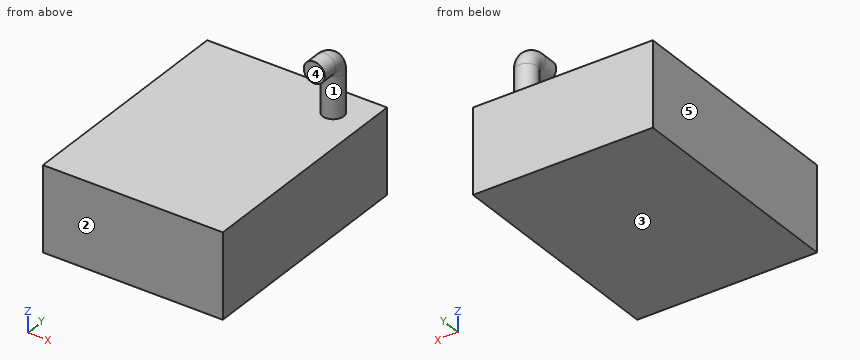
Autodesk Inventor part; units mm, degrees
ref_plane "Work Plane1" through (-215.9, 177.6349, 0) normal (0, 1, 0) x (1, 0, 0)
ref_plane "Work Plane2" through (139.7, -280.9875, 0) normal (1, 0, 0) x (0, 0, -1)
ref_plane "YZ Plane" through (0, 0, 0) normal (1, 0, 0) x (0, 1, 0)
sketch "Sketch1" plane through (0, 0, 0) normal (0, 0, 1) x (1, 0, 0)
  line L0 (215.9, -280.9875) -> (-215.9, -280.9875)
  line L1 (-215.9, -280.9875) -> (-215.9, 280.9875)
  line L2 (-215.9, 280.9875) -> (215.9, 280.9875)
  line L3 (215.9, 280.9875) -> (215.9, -280.9875)
  line L4 (215.9, -280.9875) -> (-215.9, 280.9875) construction
  line L5 (-215.9, -280.9875) -> (215.9, 280.9875) construction
  point P0 (0, 0)
  dimension "d0" = 431.8
  dimension "d1" = 561.975
extrude "Extrusion1" add sketch "Sketch1" along normal blind 203.2
sketch "Sketch2" plane through (0, 0, 203.2) normal (0, 0, 1) x (1, 0, 0)
  circle A0 centre (139.7, 205.5749) radius 25.4
  line L0 (-215.9, -280.9875) -> (215.9, -280.9875)
  line L1 (215.9, -280.9875) -> (215.9, 280.9875)
  point P0 (0, 0)
  dimension "d4" = 50.8
  dimension "d5" = 486.5624
  dimension "d6" = 76.2
extrude "Extrusion2" add sketch "Sketch2" along normal blind 98.044
ref_plane "Work Plane1" through (-215.9, 177.6349, 0) normal (0, 1, 0) x (1, 0, 0)
sketch "Sketch3" plane through (-215.9, 177.6349, 0) normal (0, 1, 0) x (1, 0, 0)
  circle A0 centre (355.6, -329.184) radius 25.4
  line L0 (330.2, -301.244) -> (381, -301.244)
  point P0 (215.9, 0)
  dimension "d16" = 27.94
extrude "Extrusion3" add sketch "Sketch3" against normal blind 36.83
ref_plane "Work Plane2" through (139.7, -280.9875, 0) normal (1, 0, 0) x (0, 0, -1)
sketch "Sketch5" plane through (0, 0, 301.244) normal (0, 0, 1) x (1, 0, 0)
  circle A0 centre (139.7, 205.5749) radius 25.4
  circle A1 centre (139.7, 205.5749) radius 25.4
  line L0 (165.1, 177.6349) -> (114.3, 177.6349)
  line L1 (114.3, 177.6349) -> (165.1, 177.6349)
  point P0 (0, 0)
revolve "Revolution1" add sketch "Sketch5" angle 90 about axis through (165.1, 177.6349, 301.244) along (1, 0, 0)
properties part number "Sump_1SDB_Tub"
Read the model definition and answer for the solid it produces. Units are mm, in the model's axes. Face numbers are marked on the shaded views. A direction names the side the tool comes from. Give positions to 0.01 mm unless a question says otherwise; leave off trailing zeros. Write each loop counter-clockwise with the first axis right and the second up, starting at its lowest first coordinate (ties: lowest second). Pieces come first, ordered by that corner, then holes. Notation, with made-up numbers: (26, 74.5) -> (51, 74.5) arc R13 ccw to (51, 98.5) -> close; hole circle Ø6 at (31.5, -12.75). An arc over 180 degrees is marked (long way). Answer as a JSON object with one key per item and string values.
1) Section C-C on y = 160.5 is taken. Write down the section's boundary in (x, z), then the cut area to 3 significant figures.
Findings below:
{"outline": "(-215.9, 0) -> (215.9, 0) -> (215.9, 203.2) -> (-215.9, 203.2) -> close; circle Ø50.8 at (139.7, 329.18)", "area": "89,800 mm^2"}
2) Straight lines are drawn through the part: probe 1 along Z at (x, y) = (-72, 81); probe 2 along Y at (x, z) = (149, 214). For each, find the intervals that lie inside material, in ascending order. Write a range as from..to.
Findings below:
{"probe 1": "z = 0..203.2", "probe 2": "y = 181.94..229.21"}
3) Section B-B on y = -131.5 is taken. Write down the section's boundary in (x, z).
Findings below:
{"outline": "(-215.9, 0) -> (215.9, 0) -> (215.9, 203.2) -> (-215.9, 203.2) -> close"}
4) Flat-ended cylindrical pins translate along their axes: pin 1 Ø8 at (x, y) = (60.5, 93) entering from +Z; pin 2 Ø15 at (x, z) = (143, 341) entering from -Y. Find the tip coordinate at first contact, or state that the pin passes through.
Findings below:
{"pin 1": "stops at z = 203.2", "pin 2": "stops at y = 140.8"}
5) Section D-D on z = 279.5 is taken. Write down the section's boundary in (x, y).
Findings below:
{"outline": "circle Ø50.8 at (139.7, 205.57)"}
6) A tool of negligible diameter and unlimited length cuts with its end or side. For the marked faces 4 and 5, from which of +Z, -Z, +X, -X, +Y, -Y can it reach the whole face along a straight path? Write none if from no direction.
Findings below:
{"face 4": "+Z, +X, -X, -Y", "face 5": "+Z, -Z, -X, +Y, -Y"}
7) Section A-A on x = 139.7 is taken. Write down the section's boundary in (y, z).
Findings below:
{"outline": "(-280.99, 0) -> (280.99, 0) -> (280.99, 203.2) -> (230.97, 203.2) -> (230.97, 301.24) arc R53.34 ccw to (177.63, 354.58) -> (140.8, 354.58) -> (140.8, 303.78) -> (177.63, 303.78) arc R2.54 cw to (180.17, 301.24) -> (180.17, 203.2) -> (-280.99, 203.2) -> close"}
8) For a pull along Z with two mould halves and no side action, classify the marked faces 1, 2 and 3 as pulls with the +Z half, pulls with the -Z half, needs draft (parallel to the pull), parting line crosses it, or undercut.
Findings below:
{"face 1": "undercut", "face 2": "needs draft", "face 3": "pulls with the -Z half"}
